Autodesk Inventor part; units mm, degrees
ref_plane "YZ Plane" through (0, 0, 0) normal (1, 0, 0) x (0, 1, 0)
ref_plane "XZ Plane" through (0, 0, 0) normal (0, 1, 0) x (-1, 0, 0)
ref_plane "XY Plane" through (0, 0, 0) normal (0, 0, 1) x (1, 0, 0)
sketch "Skizze1" plane through (0, 0, 0) normal (0, 0, 1) x (1, 0, 0)
  line L0 (45, -40) -> (-45, -40)
  line L1 (-45, -40) -> (-45, 40)
  line L2 (-45, 40) -> (45, 40)
  line L3 (45, 40) -> (45, -40)
  line L4 (45, -40) -> (-45, 40) construction
  line L5 (-45, -40) -> (45, 40) construction
  point P0 (0, 0)
  dimension "d0" = 90
  dimension "d1" = 80
extrude "Extrusion1" add sketch "Skizze1" along normal blind 1
sketch "Skizze2" plane through (0, 0, 1) normal (0, 0, 1) x (1, 0, 0)
  line L0 (-45, 40) -> (-45, -40)
  line L1 (-45, -40) -> (45, -40)
  point P0 (-5, 0)
  dimension "d13" = 40
  dimension "d23" = 40
hole "Bohrung1" at (-5, 0, 1) direction (0, 0, -1) diameter 30 end through all
sketch "Skizze3" plane through (0, 0, 1) normal (0, 0, 1) x (1, 0, 0)
  circle A0 centre (-5, 0) radius 15
  line L0 (30, 35) -> (-40, 35)
  line L1 (-40, 35) -> (-40, -35)
  line L2 (-40, -35) -> (30, -35)
  line L3 (30, -35) -> (30, 35)
  line L4 (30, 35) -> (-40, -35) construction
  line L5 (-40, 35) -> (30, -35) construction
  point P0 (0, 0)
  dimension "d14" = 70
hole "Bohrung2" at (30, -35, 1) at (-40, -35, 1) at (-40, 35, 1) at (30, 35, 1) direction (0, 0, -1) diameter 4.5 end through all
properties part number "Tunel_BackCoverToOdourPort" material "Edelstahl"
Read the model definition and answer for the solid it produces. Units are mm, in the model's axes. Coordinates: 2 decimals unless noted, no trailing zeros. Loops run counter-clockwise (first coordinate to the right, second up) from the corner with the lowest first, then second, coordinate; pieces in that order, holes last.
Q1. Consider probe 1 along X at (y, z) = (-35, 0.3); probe 2 along Y at (x, z) = (30, 0.75); probe 3 along X at (y, z) = (0, 0.2). Determine where each line is inside the solid, lowest interval first.
Q2. The part is cut by section D-D on x = 1. Write down the section's boundary in (y, z), and give its area (3 significant figures).
Q3. The part is cut by section C-C on x = 30. Write down the section's boundary in (y, z), and give its area (3 significant figures).
Q4. The part is cut by section A-A on y = 0. Write down the section's boundary in (x, z), and give its area (3 significant figures).
Q5. The mould has two halves that part along Y. Classify faces 1 (the face through (30.86, 32.92, 0.49)), 2 (the face through (9, -8, 0)): +Y half, -Y half, draft (parallel to the pull), parting line (faces both ways), or undercut.
Q6. The part is cut by section B-B on y = -35. Write down the section's boundary in (x, z).
Results below:
1. probe 1: x = -45 to -42.25, -37.75 to 27.75, 32.25 to 45
1. probe 2: y = -40 to -37.25, -32.75 to 32.75, 37.25 to 40
1. probe 3: x = -45 to -20, 10 to 45
2. outline: (-40, 0) - (-13.75, 0) - (-13.75, 1) - (-40, 1) - close; (13.75, 0) - (40, 0) - (40, 1) - (13.75, 1) - close
2. area: 52.5 mm2
3. outline: (-40, 0) - (-37.25, 0) - (-37.25, 1) - (-40, 1) - close; (-32.75, 0) - (32.75, 0) - (32.75, 1) - (-32.75, 1) - close; (37.25, 0) - (40, 0) - (40, 1) - (37.25, 1) - close
3. area: 71.0 mm2
4. outline: (-45, 0) - (-20, 0) - (-20, 1) - (-45, 1) - close; (10, 0) - (45, 0) - (45, 1) - (10, 1) - close
4. area: 60.0 mm2
5. face 1: undercut
5. face 2: draft
6. outline: (-45, 0) - (-42.25, 0) - (-42.25, 1) - (-45, 1) - close; (-37.75, 0) - (27.75, 0) - (27.75, 1) - (-37.75, 1) - close; (32.25, 0) - (45, 0) - (45, 1) - (32.25, 1) - close
